```python
from build123d import *

# Parameters (mm, degrees)
SKETCH1_W           = 50.8
SKETCH1_H           = 25.4
SKETCH1_W_2         = 44.45
SKETCH1_H_2         = 19.05
BOSS_EXTRUDE1_DEPTH = 177.8
CUT_EXTRUDE1_REACH  = 27.4
SKETCH2_R           = 2.4892
SKETCH3_R           = 2.4892
CUT_EXTRUDE2_DEPTH  = 51.8
SKETCH4_R           = 2.4892
CUT_EXTRUDE3_DEPTH  = 26.4
SKETCH5_R           = 12.7
CUT_EXTRUDE4_DEPTH  = 26.4


with BuildPart() as part:
    # Sketch1 → Boss-Extrude1 (new body, symmetric)
    with BuildSketch(Plane.XY):
        Rectangle(SKETCH1_W, SKETCH1_H)
        Rectangle(SKETCH1_W_2, SKETCH1_H_2, mode=Mode.SUBTRACT)
    extrude(amount=BOSS_EXTRUDE1_DEPTH, both=True)

    # Sketch2 → Cut-Extrude1 (cut, up to next)
    with BuildSketch(Plane.XZ.offset(-12.7), mode=Mode.PRIVATE) as cut_extrude1_sk1:
        with Locations((-12.7, 165.1)):
            Circle(SKETCH2_R)
    cut_extrude1_tool1 = extrude(cut_extrude1_sk1.sketch, amount=CUT_EXTRUDE1_REACH, mode=Mode.PRIVATE) & part.part
    add(cut_extrude1_tool1.solids().sort_by_distance((-12.7, 12.7, 165.1))[0], mode=Mode.SUBTRACT)
    # Sketch2 → Cut-Extrude1 (cut, up to next)
    with BuildSketch(Plane.XZ.offset(-12.7), mode=Mode.PRIVATE) as cut_extrude1_sk2:
        with Locations((-12.7, 152.4)):
            Circle(SKETCH2_R)
    cut_extrude1_tool2 = extrude(cut_extrude1_sk2.sketch, amount=CUT_EXTRUDE1_REACH, mode=Mode.PRIVATE) & part.part
    add(cut_extrude1_tool2.solids().sort_by_distance((-12.7, 12.7, 152.4))[0], mode=Mode.SUBTRACT)
    # Sketch2 → Cut-Extrude1 (cut, up to next)
    with BuildSketch(Plane.XZ.offset(-12.7), mode=Mode.PRIVATE) as cut_extrude1_sk3:
        with Locations((-12.7, 139.7)):
            Circle(SKETCH2_R)
    cut_extrude1_tool3 = extrude(cut_extrude1_sk3.sketch, amount=CUT_EXTRUDE1_REACH, mode=Mode.PRIVATE) & part.part
    add(cut_extrude1_tool3.solids().sort_by_distance((-12.7, 12.7, 139.7))[0], mode=Mode.SUBTRACT)
    # Sketch2 → Cut-Extrude1 (cut, up to next)
    with BuildSketch(Plane.XZ.offset(-12.7), mode=Mode.PRIVATE) as cut_extrude1_sk4:
        with Locations((-12.7, 127)):
            Circle(SKETCH2_R)
    cut_extrude1_tool4 = extrude(cut_extrude1_sk4.sketch, amount=CUT_EXTRUDE1_REACH, mode=Mode.PRIVATE) & part.part
    add(cut_extrude1_tool4.solids().sort_by_distance((-12.7, 12.7, 127))[0], mode=Mode.SUBTRACT)
    # Sketch2 → Cut-Extrude1 (cut, up to next)
    with BuildSketch(Plane.XZ.offset(-12.7), mode=Mode.PRIVATE) as cut_extrude1_sk5:
        with Locations((-12.7, 114.3)):
            Circle(SKETCH2_R)
    cut_extrude1_tool5 = extrude(cut_extrude1_sk5.sketch, amount=CUT_EXTRUDE1_REACH, mode=Mode.PRIVATE) & part.part
    add(cut_extrude1_tool5.solids().sort_by_distance((-12.7, 12.7, 114.3))[0], mode=Mode.SUBTRACT)
    # Sketch2 → Cut-Extrude1 (cut, up to next)
    with BuildSketch(Plane.XZ.offset(-12.7), mode=Mode.PRIVATE) as cut_extrude1_sk6:
        with Locations((-12.7, 101.6)):
            Circle(SKETCH2_R)
    cut_extrude1_tool6 = extrude(cut_extrude1_sk6.sketch, amount=CUT_EXTRUDE1_REACH, mode=Mode.PRIVATE) & part.part
    add(cut_extrude1_tool6.solids().sort_by_distance((-12.7, 12.7, 101.6))[0], mode=Mode.SUBTRACT)
    # Sketch2 → Cut-Extrude1 (cut, up to next)
    with BuildSketch(Plane.XZ.offset(-12.7), mode=Mode.PRIVATE) as cut_extrude1_sk7:
        with Locations((-12.7, 88.9)):
            Circle(SKETCH2_R)
    cut_extrude1_tool7 = extrude(cut_extrude1_sk7.sketch, amount=CUT_EXTRUDE1_REACH, mode=Mode.PRIVATE) & part.part
    add(cut_extrude1_tool7.solids().sort_by_distance((-12.7, 12.7, 88.9))[0], mode=Mode.SUBTRACT)
    # Sketch2 → Cut-Extrude1 (cut, up to next)
    with BuildSketch(Plane.XZ.offset(-12.7), mode=Mode.PRIVATE) as cut_extrude1_sk8:
        with Locations((12.7, 165.1)):
            Circle(SKETCH2_R)
    cut_extrude1_tool8 = extrude(cut_extrude1_sk8.sketch, amount=CUT_EXTRUDE1_REACH, mode=Mode.PRIVATE) & part.part
    add(cut_extrude1_tool8.solids().sort_by_distance((12.7, 12.7, 165.1))[0], mode=Mode.SUBTRACT)
    # Sketch2 → Cut-Extrude1 (cut, up to next)
    with BuildSketch(Plane.XZ.offset(-12.7), mode=Mode.PRIVATE) as cut_extrude1_sk9:
        with Locations((12.7, 152.4)):
            Circle(SKETCH2_R)
    cut_extrude1_tool9 = extrude(cut_extrude1_sk9.sketch, amount=CUT_EXTRUDE1_REACH, mode=Mode.PRIVATE) & part.part
    add(cut_extrude1_tool9.solids().sort_by_distance((12.7, 12.7, 152.4))[0], mode=Mode.SUBTRACT)
    # Sketch2 → Cut-Extrude1 (cut, up to next)
    with BuildSketch(Plane.XZ.offset(-12.7), mode=Mode.PRIVATE) as cut_extrude1_sk10:
        with Locations((12.7, 139.7)):
            Circle(SKETCH2_R)
    cut_extrude1_tool10 = extrude(cut_extrude1_sk10.sketch, amount=CUT_EXTRUDE1_REACH, mode=Mode.PRIVATE) & part.part
    add(cut_extrude1_tool10.solids().sort_by_distance((12.7, 12.7, 139.7))[0], mode=Mode.SUBTRACT)
    # Sketch2 → Cut-Extrude1 (cut, up to next)
    with BuildSketch(Plane.XZ.offset(-12.7), mode=Mode.PRIVATE) as cut_extrude1_sk11:
        with Locations((12.7, 127)):
            Circle(SKETCH2_R)
    cut_extrude1_tool11 = extrude(cut_extrude1_sk11.sketch, amount=CUT_EXTRUDE1_REACH, mode=Mode.PRIVATE) & part.part
    add(cut_extrude1_tool11.solids().sort_by_distance((12.7, 12.7, 127))[0], mode=Mode.SUBTRACT)
    # Sketch2 → Cut-Extrude1 (cut, up to next)
    with BuildSketch(Plane.XZ.offset(-12.7), mode=Mode.PRIVATE) as cut_extrude1_sk12:
        with Locations((12.7, 114.3)):
            Circle(SKETCH2_R)
    cut_extrude1_tool12 = extrude(cut_extrude1_sk12.sketch, amount=CUT_EXTRUDE1_REACH, mode=Mode.PRIVATE) & part.part
    add(cut_extrude1_tool12.solids().sort_by_distance((12.7, 12.7, 114.3))[0], mode=Mode.SUBTRACT)
    # Sketch2 → Cut-Extrude1 (cut, up to next)
    with BuildSketch(Plane.XZ.offset(-12.7), mode=Mode.PRIVATE) as cut_extrude1_sk13:
        with Locations((12.7, 101.6)):
            Circle(SKETCH2_R)
    cut_extrude1_tool13 = extrude(cut_extrude1_sk13.sketch, amount=CUT_EXTRUDE1_REACH, mode=Mode.PRIVATE) & part.part
    add(cut_extrude1_tool13.solids().sort_by_distance((12.7, 12.7, 101.6))[0], mode=Mode.SUBTRACT)
    # Sketch2 → Cut-Extrude1 (cut, up to next)
    with BuildSketch(Plane.XZ.offset(-12.7), mode=Mode.PRIVATE) as cut_extrude1_sk14:
        with Locations((12.7, 88.9)):
            Circle(SKETCH2_R)
    cut_extrude1_tool14 = extrude(cut_extrude1_sk14.sketch, amount=CUT_EXTRUDE1_REACH, mode=Mode.PRIVATE) & part.part
    add(cut_extrude1_tool14.solids().sort_by_distance((12.7, 12.7, 88.9))[0], mode=Mode.SUBTRACT)

    # Sketch3 → Cut-Extrude2 (cut, through all)
    with BuildSketch(Plane(origin=(25.4, 0, 0), x_dir=(0, 0, -1), z_dir=(1, 0, 0))):
        with Locations((-165.1, 0)):
            Circle(SKETCH3_R)
        with Locations((-139.7, 0)):
            Circle(SKETCH3_R)
        with Locations((-114.3, 0)):
            Circle(SKETCH3_R)
        with Locations((-88.9, 0)):
            Circle(SKETCH3_R)
        with Locations((-63.5, 0)):
            Circle(SKETCH3_R)
        with Locations((-38.1, 0)):
            Circle(SKETCH3_R)
        with Locations((-12.7, 0)):
            Circle(SKETCH3_R)
        with Locations((12.7, 0)):
            Circle(SKETCH3_R)
        with Locations((38.1, 0)):
            Circle(SKETCH3_R)
        with Locations((63.5, 0)):
            Circle(SKETCH3_R)
        with Locations((88.9, 0)):
            Circle(SKETCH3_R)
        with Locations((114.3, 0)):
            Circle(SKETCH3_R)
        with Locations((139.7, 0)):
            Circle(SKETCH3_R)
        with Locations((165.1, 0)):
            Circle(SKETCH3_R)
    extrude(amount=-CUT_EXTRUDE2_DEPTH, mode=Mode.SUBTRACT)

    # Sketch4 → Cut-Extrude3 (cut, through all)
    with BuildSketch(Plane.XZ.offset(12.7)):
        with Locations((-12.7, -152.4)):
            Circle(SKETCH4_R)
        with Locations((-12.7, -139.7)):
            Circle(SKETCH4_R)
        with Locations((-12.7, -127)):
            Circle(SKETCH4_R)
        with Locations((-12.7, -114.3)):
            Circle(SKETCH4_R)
        with Locations((-12.7, -101.6)):
            Circle(SKETCH4_R)
        with Locations((-12.7, -88.9)):
            Circle(SKETCH4_R)
        with Locations((-12.7, -76.2)):
            Circle(SKETCH4_R)
        with Locations((-12.7, -63.5)):
            Circle(SKETCH4_R)
        with Locations((-12.7, -50.8)):
            Circle(SKETCH4_R)
        with Locations((12.7, -50.8)):
            Circle(SKETCH4_R)
        with Locations((12.7, -63.5)):
            Circle(SKETCH4_R)
        with Locations((12.7, -76.2)):
            Circle(SKETCH4_R)
        with Locations((12.7, -88.9)):
            Circle(SKETCH4_R)
        with Locations((12.7, -101.6)):
            Circle(SKETCH4_R)
        with Locations((12.7, -114.3)):
            Circle(SKETCH4_R)
        with Locations((12.7, -127)):
            Circle(SKETCH4_R)
        with Locations((12.7, -139.7)):
            Circle(SKETCH4_R)
        with Locations((12.7, -152.4)):
            Circle(SKETCH4_R)
    extrude(amount=-CUT_EXTRUDE3_DEPTH, mode=Mode.SUBTRACT)

    # Sketch5 → Cut-Extrude4 (cut, through all)
    with BuildSketch(Plane(origin=(0, 12.7, 0), x_dir=(1, 0, 0), z_dir=(0, 1, 0))):
        with Locations((0, -57.15)):
            Circle(SKETCH5_R)
        with Locations((0, -19.05)):
            Circle(SKETCH5_R)
        with Locations((0, 19.05)):
            Circle(SKETCH5_R)
    extrude(amount=-CUT_EXTRUDE4_DEPTH, mode=Mode.SUBTRACT)


solid = part.part
```
Verification items for the finished model (mm, model axes). A direction names the side the tool comes from. Round coordinates to 2 decimals unless told otherwise and drop trailing zeros. Order: outer loops, then holes, each group sorted by start corner. A loop starts at its lowest first (then second) coordinate and runs counter-clockwise, first axis right, second up. Notation, with made-up numbers: (13, 81) -> (44, 81) arc R35 cw to (44, 118) -> close; hole circle Ø4 at (44, 73.5). An arc over 180 degrees is marked (long way). Put each result on its own line as item: value. Start each with the question number.
(1) Section check B-B (z = -58). Enter the section's corners in (x, y) (3 decimals).
(2) Material ranges on line 1 along X through (y, z) = (11.9, 88.9); line 2 along Y through (x, z) = (-15, 36.5) (3 decimals); line 3 along X through (y, z) = (0.5, -66) (3 decimals), recorded low to high.
(3) Section check C-C (x = 1.5). State how many separate pieces and enclosed holes the cut face has, then the cut area to 3 significant figures.
(4) Depth check by flat-ended pin: pin 1 Ø4.5 at (y, z) = (0, 38.1) entering from -X; pin 2 Ø3 at (x, z) = (12.7, 88.9) entering from +Y (3 decimals). Enter the tip coordinate at first touch or a pass-through.
(5) Section check A-A (y = 6.5). Enter the section's corners in (x, z) (3 decimals), then the cut area to 3 significant figures.
(6) Section check D-D (z = 57.15). Enter the section's corners in (x, y) (3 decimals), then the cut area to 3 significant figures.
(7) Tool access check on faces 4 (the face through (-1.653, 11.135, 44.558)), 5 (the face through (0, -9.525, 2)). Record the directions out of +Z, -Z, +X, -X, +Y, -Y that give a thin tool (end or side, any length) a straight path to the whole face; none if there is none.
(8) Draft check along Z on faces 1 (the face through (0, 12.7, 2)), 2 (the face through (0, 10, -177.8)), 3 (the face through (-1.653, -11.09, 6.458)). Enter one of: +Z half, -Z half, draft (parallel to the pull), parting line (faces both ways), or undercut.
Completed:
1. outline: (-25.4, -12.7) -> (25.4, -12.7) -> (25.4, 12.7) -> (-25.4, 12.7) -> close; hole (-22.225, -9.525) -> (22.225, -9.525) -> (22.225, 9.525) -> (-22.225, 9.525) -> close
2. line 1: x = -25.4 to -15.19, -10.21 to 10.21, 15.19 to 25.4
2. line 2: y = -12.7 to -9.525, 9.525 to 12.7
2. line 3: x = -25.4 to -22.225, 22.225 to 25.4
3. separate pieces: 8
3. enclosed holes: 0
3. area: 1,780 mm2
4. pin 1: passes through
4. pin 2: stops at y = -9.525
5. outline: (-25.4, -177.8) -> (-22.225, -177.8) -> (-22.225, 177.8) -> (-25.4, 177.8) -> close; (22.225, -177.8) -> (25.4, -177.8) -> (25.4, 177.8) -> (22.225, 177.8) -> close
5. area: 2,260 mm2
6. outline: (-25.4, -12.7) -> (-12.7, -12.7) -> (-12.7, -9.525) -> (-22.225, -9.525) -> (-22.225, 9.525) -> (-12.7, 9.525) -> (-12.7, 12.7) -> (-25.4, 12.7) -> close; (12.7, -12.7) -> (25.4, -12.7) -> (25.4, 12.7) -> (12.7, 12.7) -> (12.7, 9.525) -> (22.225, 9.525) -> (22.225, -9.525) -> (12.7, -9.525) -> close
6. area: 282 mm2
7. face 4: +Y, -Y
7. face 5: +Z, -Z
8. face 1: draft
8. face 2: -Z half
8. face 3: undercut
